Verification items for this drawing (mm, ordinates from the low corner). A direction names the side the tool comes from. Give positions to 0.01 mm unless a question says otherwise; leave off trailing zeros. Loops run counter-clockwise (first coordinate to the right, second up) from the corner with the lowest first, then second, coordinate; pieces in that order, holes last. Notation, with made-up numbers: (21.5, 55) - (72.5, 55) arc R21 ccw to (72.5, 74) - close; hole circle Ø7 at (75.25, -3.5). An arc over 180 degrees is marked (long way). Write item = value, one per line. Start each with the question number.
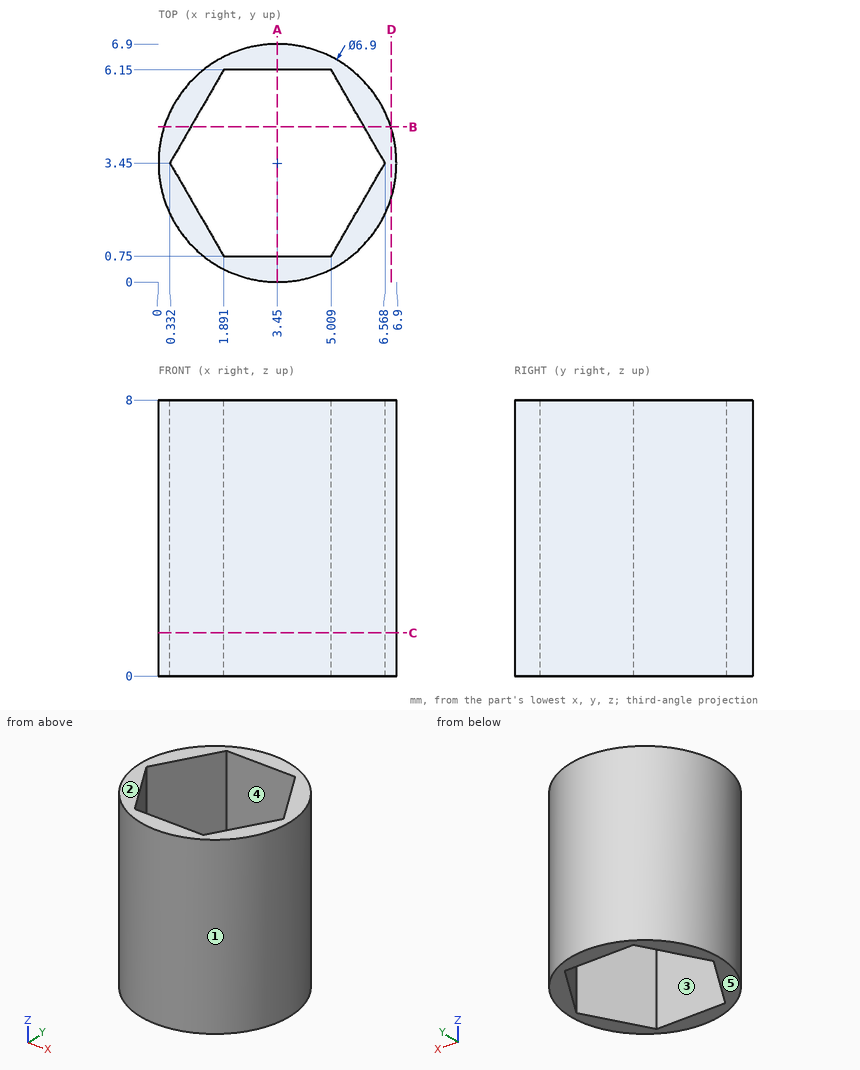
1) Release check for a two-part mould opening along Y. For the marked faces 1, 2 and 3 record: pulls with the +Y half, pulls with the -Y half, needs draft (parallel to the pull), parting line crosses it, or undercut.
2) Cross-section at B-B on y = 4.5. Enter the section's corners in (x, z), and give its area (3 significant figures).
3) Cross-section at C-C on z = 1.25. Enter the section's corners in (x, y).
4) Cross-section at A-A on x = 3.45. Enter the section's corners in (y, z), and give its area (3 significant figures).
5) Cross-section at D-D on x = 6.75. Enter the section's corners in (y, z).
6) Material ranges on line 1 along Y through (x, z) = (3.5, 5.5); line 2 along Y through (x, z) = (5.5, 4) (1 decimal); line 3 along X through (y, z) = (1.5, 6) (1 decimal), recorded low to high.
7) Tool access check on the marked faces 4 and 5. Record the directions out of +Z, -Z, +X, -X, +Y, -Y that give a thin tool (end or side, any length) a straight path to the whole face; none if there is none.
8) Gauge pin test, flat ends, axial feed: P1, Ø4, axis at x = 6, z = 6, coming from the -Y side; P2, Ø2, axis at x = 6, z = 2.5, coming from the -Y side. Record the tip position at first contact, or that the pin passes through.
Checked values:
q1.face_1 = parting line crosses it
q1.face_2 = needs draft
q1.face_3 = undercut
q2.outline = (0.16, 0) - (0.94, 0) - (0.94, 8) - (0.16, 8) - close; (5.96, 0) - (6.74, 0) - (6.74, 8) - (5.96, 8) - close
q2.area = 12.4 mm²
q3.outline = circle Ø6.9 at (3.45, 3.45); hole (0.33, 3.45) - (1.89, 0.75) - (5.01, 0.75) - (6.57, 3.45) - (5.01, 6.15) - (1.89, 6.15) - close
q4.outline = (0, 0) - (0.75, 0) - (0.75, 8) - (0, 8) - close; (6.15, 0) - (6.9, 0) - (6.9, 8) - (6.15, 8) - close
q4.area = 12.0 mm²
q5.outline = (2.44, 0) - (4.46, 0) - (4.46, 8) - (2.44, 8) - close
q6.line_1 = 0 to 0.75, 6.15 to 6.9
q6.line_2 = 0.7 to 1.6, 5.3 to 6.2
q6.line_3 = 0.6 to 1.5, 5.4 to 6.3
q7.face_4 = +Z, -Z
q7.face_5 = -Z, +X, -X, +Y, -Y
q8.P1 = 0.04
q8.P2 = 0.37
